from build123d import *

# Parameters (mm, degrees)
F1_DEPTH = 17.78
F2_W     = 7.62
F2_H     = 17.78
F3_DEPTH = 16.51
F4_SIZE  = 6.35
F5_R     = 2.65
F6_DEPTH = 25.4
F7_R     = 2.794
F8_R     = 5.08
F9_R     = 5.08
F10_R    = 5.08
F11_R    = 5.08


# Not quite as in the source:
# - a feature names something its author has since deleted; it is built from what else it names


with BuildPart() as f1:
    # F0 (on Top) → F1 (new body)
    with BuildSketch(Plane.XY):
        Polygon((5.5632305153, 1.0289779667), (5.5632305153, -11.6080572072), (3.1819805153, -11.6080572072), (0, -8.4260766918), (-3.1819805153, -11.6080572072), (-3.1819805153, -17.9580572072), (13.6277864288, -17.9580572072), (13.6277864288, -1.148290263), (6.8148051953, 5.6646909705), (-0.4051948047, 5.6646909705), (-3.1819805153, 5.6646909705), (-3.1819805153, 1.0289779667), (0, -2.1530025487), (3.1819805153, 1.0289779667), align=None)
    extrude(amount=F1_DEPTH)

    # F2 (on face) → F3 (join)
    with BuildSketch(Plane.YZ.offset(13.6277864288)):
        with Locations((-4.958290263, 8.89)):
            Rectangle(F2_W, F2_H)
    extrude(amount=F3_DEPTH)

    # F4
    f4_edges = [f1.edges().sort_by_distance(p)[0] for p in [
        (30.137786, -4.95829, 17.78),
    ]]
    chamfer(f4_edges, length=F4_SIZE)

    # F5 (on face) → F6 (cut)
    with BuildSketch(Plane.XZ.offset(8.768290263)):
        with Locations((23.1527864288, 6.35)):
            Circle(F5_R)
    extrude(amount=-F6_DEPTH, mode=Mode.SUBTRACT)

    # F7
    f7_edges = [f1.edges().sort_by_distance(p)[0] for p in [
        (0, -8.426077, 8.89),
    ]]
    fillet(f7_edges, radius=F7_R)

    # F8
    f8_edges = [f1.edges().sort_by_distance(p)[0] for p in [
        (6.814805, 5.664691, 8.89),
    ]]
    fillet(f8_edges, radius=F8_R)

    # F9
    f9_edges = [f1.edges().sort_by_distance(p)[0] for p in [
        (30.137786, -4.95829, 0),
    ]]
    fillet(f9_edges, radius=F9_R)

    # F10
    f10_edges = [f1.edges().sort_by_distance(p)[0] for p in [
        (13.627786, -17.958057, 8.89),
    ]]
    fillet(f10_edges, radius=F10_R)

    # F11
    f11_edges = [f1.edges().sort_by_distance(p)[0] for p in [
        (30.137786, -4.95829, 11.43),
        (23.787786, -4.95829, 17.78),
    ]]
    fillet(f11_edges, radius=F11_R)


solid = f1.part
CAD build for the part. Positions are in the model's coordinates, mm. A direction names the side the tool comes from. Coordinates: 2 decimals unless noted, no trailing zeros. Write each loop counter-clockwise with the first axis right and the second up, starting at its lowest first coordinate (ties: lowest second). Pieces come first, ordered by that corner, then holes. Notation, with made-up numbers: M 89,-14 L 99,-14 A12 cw 99,7 Z; hole C 57,60.5 d5. An arc over 180 degrees is marked long. Answer as a JSON object with one key per item and string values. Group by question number.
1) Wall check: line 1 (X direction, y = -2, z = 5); line 2 (X direction, y = -1.5, z = 5.75); line 3 (Y direction, x = 23.5, z = 16). Give the ranges that are in metal, low to high. Write a range as from..to.
2) Saw through at B-B (z = 6.35). Write the cut outline in (x, y).
3) Mould opens along X. For faces 5 (the face through (4, -11.608, 9)), 6 (the face through (13.628, -11, 9)), 7 (the face through (22, -8.768, 9)) say: +X half, -X half, draft (parallel to the pull), parting line (faces both ways), or undercut.
4) Saw through at C-C (y = -4). Write the cut outline in (x, z).
5) Tool access for faces 1 (the face through (22, -1.148, 9)), 2 (the face through (-0.031, -9.584, 9.014)), 3 (the face through (8, -6, 0)), 4 (the face through (-2.57, -10.996, 8.766)): list every direction of +Z, -Z, +X, -X, +Y, -Y with a clear straight run to the whole face (end or side of a thin tool).
6) Saw through at A-A (x = 4). Write the cut outline in (y, z).
7) Saw through at D-D (z = 3.25). Write the cut outline in (x, y).
8) Pin check, flat tips, straight feed: pin 1 Ø5 at (y, z) = (-11.5, 14.5) entering from +X; pin 2 Ø3 at (x, z) = (23.15, 6.35) entering from -Y; pin 3 Ø2 at (x, y) = (7, -11) entering from -Z; pin 4 Ø5 at (y, z) = (-3, 14.5) entering from +X. Stop position of each tip, or through.
Values follow:
{
 "1": {"line 1": "x = -0.15..0.15, 5.56..20.87, 25.43..30.14", "line 2": "x = -0.65..0.65, 5.56..20.57, 25.73..30.14", "line 3": "y = -8.77..-1.15"},
 "2": {"outline": "M -3.18,-17.96 L 8.55,-17.96 A5.08 ccw 13.63,-12.88 L 13.63,-8.77 L 20.5,-8.77 L 20.5,-1.15 L 13.63,-1.15 L 8.3,4.18 A5.08 ccw 4.71,5.66 L -3.18,5.66 L -3.18,1.03 L 0,-2.15 L 3.18,1.03 L 5.56,1.03 L 5.56,-11.61 L 3.18,-11.61 L 1.98,-10.4 A2.79 ccw -1.98,-10.4 L -3.18,-11.61 Z; M 25.8,-8.77 L 30.14,-8.77 L 30.14,-1.15 L 25.8,-1.15 Z"},
 "3": {"face 5": "undercut", "face 6": "+X half", "face 7": "draft"},
 "4": {"outline": "M 5.56,0 L 25.06,0 A5.08 ccw 30.14,5.08 L 30.14,9.33 A5.08 ccw 28.65,12.92 L 25.28,16.29 A5.08 ccw 21.68,17.78 L 5.56,17.78 Z; hole C 23.15,6.35 d5.3"},
 "5": {"face 1": "+Z, -Z, +X, +Y", "face 2": "+Z, -Z", "face 3": "-Z, +X, -X, +Y, -Y", "face 4": "+Z, -Z, -X"},
 "6": {"outline": "M -17.96,0 L -11.61,0 L -11.61,17.78 L -17.96,17.78 Z; M 1.03,0 L 5.66,0 L 5.66,17.78 L 1.03,17.78 Z"},
 "7": {"outline": "M -3.18,-17.96 L 8.55,-17.96 A5.08 ccw 13.63,-12.88 L 13.63,-8.77 L 29.8,-8.77 L 29.8,-1.15 L 13.63,-1.15 L 8.3,4.18 A5.08 ccw 4.71,5.66 L -3.18,5.66 L -3.18,1.03 L 0,-2.15 L 3.18,1.03 L 5.56,1.03 L 5.56,-11.61 L 3.18,-11.61 L 1.98,-10.4 A2.79 ccw -1.98,-10.4 L -3.18,-11.61 Z"},
 "8": {"pin 1": "stops at x = 13.63", "pin 2": "passes through", "pin 3": "stops at z = 0", "pin 4": "stops at x = 29.38"}
}
